```python
from build123d import *

# Parameters (mm, degrees)
SALIENTE_EXTRUIR1_DEPTH = 50
CROQUIS2_W              = 50
CROQUIS2_H              = 2
SALIENTE_EXTRUIR2_DEPTH = 20


with BuildPart() as part:
    # Croquis1 → Saliente-Extruir1 (new body)
    with BuildSketch(Plane.XY):
        Polygon((-84.492533904, -6.999380213), (-44.492533904, -6.999380213), (-44.492533904, -5.738560558), (-44.492533904, -4.999380213), (-45.492533904, -4.999380213), (-57.147376638, -4.999380213), (-57.147376638, 9.072422448), (-51.585761076, 18.705423174), (-51.085761076, 19.571448577), (-54.549862691, 21.571448577), (-69.313187577, -3.999380213), (-81.019143074, -3.999380213), (-80.530687688, -2.657360069), (-77.297371662, 6.226102703), (-76.955351518, 7.165795324), (-79.774429381, 8.191855754), (-80.129339821, 7.280632657), (-84.424349875, -3.746691195), (-84.492533904, -3.921751872), (-84.492533904, -4.109622312), align=None)
    extrude(amount=SALIENTE_EXTRUIR1_DEPTH)

    # Croquis2 → Saliente-Extruir2 (add)
    with BuildSketch(Plane(origin=(-44.492533904, 0, 0), x_dir=(0, 0, -1), z_dir=(1, 0, 0))):
        with Locations((-25, -5.999380213)):
            Rectangle(CROQUIS2_W, CROQUIS2_H)
    extrude(amount=SALIENTE_EXTRUIR2_DEPTH)


solid = part.part
```
Source: CAD feature listing. Evaluate the final solid. Frame: model axes, mm. A direction names the side the tool comes from. Round coordinates to 2 decimals unless told otherwise and drop trailing zeros. Loops run counter-clockwise (first coordinate to the right, second up) from the corner with the lowest first, then second, coordinate; pieces in that order, holes last.
(1) Contact query for flat-ended pins moving along their axis: pin 1 Ø7 at (y, z) = (-1, 33) entering from +X; pin 2 Ø2 at (x, z) = (-46.5, 21) entering from +Y; pin 3 Ø16.5 at (x, z) = (-48.5, 32) entering from +Y. Output: stop coordinate, or through.
From the geometry:
pin 1: stops at x = -57.15
pin 2: stops at y = -5
pin 3: stops at y = 21.57
(2) Material intervals for probe 1 along Y at (x, z) = (-30, 29.5); probe 2 along X at (y, z) = (-1, 4); probe 3 along Y at (x, z) = (-53.5, 47.5), sorted ascending.
From the geometry:
probe 1: y = -7 to -5
probe 2: x = -83.35 to -79.93, -67.58 to -57.15
probe 3: y = -7 to -5, 15.39 to 20.97
(3) Section query B-B (y = 3.25). Output: boundary loops of the cut face in (x, z), and give its area (3 significant figures).
From the geometry:
outline: (-81.7, 0) - (-78.38, 0) - (-78.38, 50) - (-81.7, 50) - close; (-65.13, 0) - (-57.15, 0) - (-57.15, 50) - (-65.13, 50) - close
area: 565 mm2
(4) Section query C-C (x = -42). Output: boundary loops of the cut face in (y, z), and give its area (3 significant figures).
From the geometry:
outline: (-7, 0) - (-5, 0) - (-5, 50) - (-7, 50) - close
area: 100 mm2
(5) Section query D-D (y = 0). Output: boundary loops of the cut face in (x, z).
From the geometry:
outline: (-82.97, 0) - (-79.56, 0) - (-79.56, 50) - (-82.97, 50) - close; (-67, 0) - (-57.15, 0) - (-57.15, 50) - (-67, 50) - close
(6) Pull-direction query (X, two-part tool) for faces 1 (the flat face through (-84.493, -5, 25)), 2 (the flat face through (-24.493, -6, 25)), 3 (the flat face through (-55, -6.999, 25)), 4 (the flat face through (-75, -3.999, 25)); classes: +X half, -X half, draft (parallel to the pull), parting line (faces both ways), or undercut.
From the geometry:
face 1: -X half
face 2: +X half
face 3: draft
face 4: undercut
(7) Access query for faces 5 (the flat face through (-59, 1, 50)), 6 (the flat face through (-61.828, 8.965, 24.65)), 7 (the flat face through (-41, -4.999, 25)). Directions: +Z, -Z, +X, -X, +Y, -Y. A direction counts if a zero-diameter tool reaches every point of the face in a straight line with its end or side. Return the directions, or none.
From the geometry:
face 5: +Z, +X, -X, +Y, -Y
face 6: +Z, -Z, +Y
face 7: +Z, -Z, +X
(8) Section query A-A (z = 34). Output: boundary loops of the cut face in (x, y), and give its area (3 significant figures).
From the geometry:
outline: (-84.49, -7) - (-24.49, -7) - (-24.49, -5) - (-57.15, -5) - (-57.15, 9.07) - (-51.09, 19.57) - (-54.55, 21.57) - (-69.31, -4) - (-81.02, -4) - (-76.96, 7.17) - (-79.77, 8.19) - (-84.49, -3.92) - close
area: 349 mm2
